from build123d import *

# Parameters (mm, degrees)
EXTRUDE_1_DEPTH     = 3
SKETCH_2_W          = 40
SKETCH_2_H          = 3
EXTRUDE_2_DEPTH     = 40
SKETCH_3_R          = 2.6
CUT_EXTRUDE_1_DEPTH = 40
FILLET_1_R          = 3


with BuildPart() as part:
    # 草图1 → 凸台-拉伸1 (new body)
    with BuildSketch(Plane.XY):
        with BuildLine():
            Line((11, 0), (13.502586321, 0))
            ThreePointArc((13.502586321, 0), (13.915065254, 1.032067984), (14.925258409, 1.495547198))
            ThreePointArc((14.925258409, 1.495547198), (13.858192988, 5.740251485), (11.611262997, 9.496239867))
            ThreePointArc((11.611262997, 9.496239867), (9.547770351, 9.547770351), (9.496239867, 11.611262997))
            ThreePointArc((9.496239867, 11.611262997), (5.740251485, 13.858192988), (1.495547198, 14.925258409))
            ThreePointArc((1.495547198, 14.925258409), (0, 13.502586321), (-1.495547198, 14.925258409))
            ThreePointArc((-1.495547198, 14.925258409), (-6.339273926, 13.594616806), (-10.472092058, 10.739426797))
            ThreePointArc((-10.472092058, 10.739426797), (-10.118173432, 10.240571276), (-9.993252967, 9.641814145))
            ThreePointArc((-9.993252967, 9.641814145), (-10.824149511, 8.300917939), (-12.394730475, 8.448115556))
            ThreePointArc((-12.394730475, 8.448115556), (-14.095389312, 5.13030215), (-14.925258409, 1.495547198))
            ThreePointArc((-14.925258409, 1.495547198), (-13.915065254, 1.032067984), (-13.502586321, 0))
            Line((-13.502586321, 0), (-11, 0))
            ThreePointArc((-11, 0), (0, 11), (11, 0))
        make_face()
        with BuildLine():
            ThreePointArc((14.925258409, -1.495547198), (13.915065254, -1.032067984), (13.502586321, 0))
            Line((13.502586321, 0), (11, 0))
            ThreePointArc((11, 0), (0, -11), (-11, 0))
            Line((-11, 0), (-13.502586321, 0))
            ThreePointArc((-13.502586321, 0), (-13.915065254, -1.032067984), (-14.925258409, -1.495547198))
            ThreePointArc((-14.925258409, -1.495547198), (-13.858192988, -5.740251485), (-11.611262997, -9.496239867))
            ThreePointArc((-11.611262997, -9.496239867), (-9.99920803, -9.237908679), (-9.109188038, -10.606601718))
            ThreePointArc((-9.109188038, -10.606601718), (-9.209297393, -11.144921652), (-9.496239867, -11.611262997))
            ThreePointArc((-9.496239867, -11.611262997), (-5.740251485, -13.858192988), (-1.495547198, -14.925258409))
            ThreePointArc((-1.495547198, -14.925258409), (0, -13.502586321), (1.495547198, -14.925258409))
            ThreePointArc((1.495547198, -14.925258409), (6.339273926, -13.594616806), (10.472092058, -10.739426797))
            ThreePointArc((10.472092058, -10.739426797), (10.343581219, -8.679295186), (12.394730475, -8.448115556))
            ThreePointArc((12.394730475, -8.448115556), (14.095389312, -5.13030215), (14.925258409, -1.495547198))
        make_face()
        with BuildLine():
            ThreePointArc((14.925258409, 1.495547198), (16.032067984, 1.084934746), (16.497413679, 0))
            Line((16.497413679, 0), (20, 0))
            ThreePointArc((20, 0), (0, 20), (-20, 0))
            Line((-20, 0), (-16.497413679, 0))
            ThreePointArc((-16.497413679, 0), (-16.032067984, 1.084934746), (-14.925258409, 1.495547198))
            ThreePointArc((-14.925258409, 1.495547198), (-14.095389312, 5.13030215), (-12.394730475, 8.448115556))
            ThreePointArc((-12.394730475, 8.448115556), (-12.637752075, 10.604333105), (-10.472092058, 10.739426797))
            ThreePointArc((-10.472092058, 10.739426797), (-6.339273926, 13.594616806), (-1.495547198, 14.925258409))
            ThreePointArc((-1.495547198, 14.925258409), (-0.037382446, 16.496946986), (1.497413679, 15))
            ThreePointArc((1.497413679, 15), (1.496946986, 14.962617554), (1.495547198, 14.925258409))
            ThreePointArc((1.495547198, 14.925258409), (5.740251485, 13.858192988), (9.496239867, 11.611262997))
            ThreePointArc((9.496239867, 11.611262997), (11.144921652, 12.003906043), (12.104015397, 10.606601718))
            ThreePointArc((12.104015397, 10.606601718), (11.975294757, 9.99920803), (11.611262997, 9.496239867))
            ThreePointArc((11.611262997, 9.496239867), (13.858192988, 5.740251485), (14.925258409, 1.495547198))
        make_face()
        with BuildLine():
            Line((20, 0), (16.497413679, 0))
            ThreePointArc((16.497413679, 0), (16.032067984, -1.084934746), (14.925258409, -1.495547198))
            ThreePointArc((14.925258409, -1.495547198), (14.095389312, -5.13030215), (12.394730475, -8.448115556))
            ThreePointArc((12.394730475, -8.448115556), (12.831562853, -8.97529701), (12.988080326, -9.641814145))
            ThreePointArc((12.988080326, -9.641814145), (12.089423778, -11.01430736), (10.472092058, -10.739426797))
            ThreePointArc((10.472092058, -10.739426797), (6.339273926, -13.594616806), (1.495547198, -14.925258409))
            ThreePointArc((1.495547198, -14.925258409), (1.496946986, -14.962617554), (1.497413679, -15))
            ThreePointArc((1.497413679, -15), (-0.037382446, -16.496946986), (-1.495547198, -14.925258409))
            ThreePointArc((-1.495547198, -14.925258409), (-5.740251485, -13.858192988), (-9.496239867, -11.611262997))
            ThreePointArc((-9.496239867, -11.611262997), (-11.665433085, -11.665433085), (-11.611262997, -9.496239867))
            ThreePointArc((-11.611262997, -9.496239867), (-13.858192988, -5.740251485), (-14.925258409, -1.495547198))
            ThreePointArc((-14.925258409, -1.495547198), (-16.032067984, -1.084934746), (-16.497413679, 0))
            Line((-16.497413679, 0), (-20, 0))
            ThreePointArc((-20, 0), (0, -20), (20, 0))
        make_face()
        with BuildLine():
            Line((20, -28), (20, 0))
            ThreePointArc((20, 0), (0, -20), (-20, 0))
            Line((-20, 0), (-20, -28))
            Line((-20, -28), (20, -28))
        make_face()
    extrude(amount=EXTRUDE_1_DEPTH)

    # 草图2 → 凸台-拉伸2 (add)
    with BuildSketch(Plane.XY.offset(3)):
        with Locations((0, -26.5)):
            Rectangle(SKETCH_2_W, SKETCH_2_H)
    extrude(amount=EXTRUDE_2_DEPTH)

    # 草图3 → 切除-拉伸1 (cut)
    with BuildSketch(Plane(origin=(0, -25, 0), x_dir=(1, 0, 0), z_dir=(0, 1, 0))):
        with Locations(Location((-15, -13, 0), (0, 0, 270))):
            Circle(SKETCH_3_R)
        with Locations(Location((-15, -33, 0), (0, 0, 270))):
            Circle(SKETCH_3_R)
        with Locations(Location((15, -33, 0), (0, 0, 270))):
            Circle(SKETCH_3_R)
        with Locations(Location((15, -13, 0), (0, 0, 270))):
            Circle(SKETCH_3_R)
    extrude(amount=-CUT_EXTRUDE_1_DEPTH, mode=Mode.SUBTRACT)

    # 圆角1
    fillet_1_edges = [part.edges().sort_by_distance(p)[0] for p in [
        (0, -28, 0),
        (-20, -26.5, 43),
        (20, -26.5, 43),
    ]]
    fillet(fillet_1_edges, radius=FILLET_1_R)


solid = part.part
Here's how the part is built. I have some questions about the finished solid (model axes, mm). A direction names the side the tool comes from. Coordinates: 2 decimals unless noted, no trailing zeros. Order: outer loops, then holes, each group sorted by start corner. A loop starts at its lowest first (then second) coordinate and runs counter-clockwise, first axis right, second up. Notation, with made-up numbers: (-22, 76) - (9, 76) arc R16 ccw to (9, 99) - close; hole circle Ø3 at (-28, 78). An arc over 180 degrees is marked (long way). Use CSV: the item, a comma, the result in double quotes. Start each with the question number.
1. I'm going to push flat-ended pins straight in: pin 1 (20 mm diameter, centred on x = -6, z = 17, fed in from +Y); pin 2 (12 mm diameter, centred on x = -6, y = 1, fed in from +Z). Where does each tip first touch, or does it pass through?
2. Suppose I cut it at B-B on x = 3. List the corners of the cut face in (y, z) for me.
3. Suppose I cut it at A-A on z = 13. List the corners of the cut face in (x, y) for me.
4. If we mould it in two halves opening along Z, with no side actions, what happens to faces 1 (the face through (14, -26.5, 15.4)), 2 (the face through (0, -12, 3)), 3 (the face through (-16, -26.5, 15.4)), 4 (the face through (-20, -25.5, 12.5))? For each: +Z half, -Z half, draft (parallel to the pull), parting line (faces both ways), or undercut.
5. For faces 5 (the face through (19.1, -26.48, 42.14)), 6 (the face through (0, -25, 23)), which set-ups out of +Z, -Z, +X, -X, +Y, -Y let a thin tool reach every point of the face, with its end or its side?
6. Please list where these lines run through material, in increasing order: line 1 (X direction, y = -26, z = 13); line 2 (Z direction, x = -14, y = -3.5); line 3 (Y direction, x = -18, z = 16.5). Write a range as from..to.
7. Suppose I cut it at D-D on z = 32. List the corners of the cut face in (x, y) for me, then the cut area to 3 significant figures.
8. Suppose I cut it at C-C on y = -6.5. List the corners of the cut face in (x, z) for me.
Output:
1,pin 1,"stops at y = -25"
1,pin 2,"stops at z = 3"
2,outline,"(-28, 3) arc R3 ccw to (-25, 0) - (-10.58, 0) - (-10.58, 3) - (-25, 3) - (-25, 43) - (-28, 43) - close; (10.58, 0) - (19.77, 0) - (19.77, 3) - (10.58, 3) - close"
3,outline,"(-20, -28) - (-17.6, -28) - (-17.6, -25) - (-20, -25) - close; (-12.4, -28) - (12.4, -28) - (12.4, -25) - (-12.4, -25) - close; (17.6, -28) - (20, -28) - (20, -25) - (17.6, -25) - close"
4,face 1,"undercut"
4,face 2,"+Z half"
4,face 3,"undercut"
4,face 4,"draft"
5,face 5,"+Z, +X, +Y, -Y"
5,face 6,"+Z, +X, -X, +Y"
6,line 1,"x = -20..-17.6, -12.4..12.4, 17.6..20"
6,line 2,"z = 0..3"
6,line 3,"y = -28..-25"
7,outline,"(-20, -28) - (-17.4, -28) - (-17.4, -25) - (-20, -25) - close; (-12.6, -28) - (12.6, -28) - (12.6, -25) - (-12.6, -25) - close; (17.4, -28) - (20, -28) - (20, -25) - (17.4, -25) - close"
7,area,"91.2 mm2"
8,outline,"(-20, 0) - (-8.87, 0) - (-8.87, 3) - (-20, 3) - close; (8.87, 0) - (20, 0) - (20, 3) - (8.87, 3) - close"
